Read the model definition and answer for the solid it produces. Units are mm, in the model's axes. A direction names the side the tool comes from. Coordinates: 2 decimals unless noted, no trailing zeros. Order: outer loops, then holes, each group sorted by start corner. A loop starts at its lowest first (then second) coordinate and runs counter-clockwise, first axis right, second up.
```python
from build123d import *

# Parameters (mm, degrees)
SKETCH11_W              = 17
SKETCH11_H              = 19.920243607
BOSS_EXTRUDE7_DEPTH     = 1
BOSS_EXTRUDE5_START     = -2.131780543
BOSS_EXTRUDE5_OUTLINE_W = 1
BOSS_EXTRUDE5_OUTLINE_H = 7
BOSS_EXTRUDE5_DEPTH     = 19.920243607
SKETCH13_W              = 1
SKETCH13_H              = 19.920243607
BOSS_EXTRUDE6_DEPTH     = 7
LPATTERN3_COUNT         = 7
LPATTERN3_PITCH         = 2
CUT_EXTRUDE1_REACH      = 23.276
SKETCH14_R              = 1.905


# Read off the part's stored shape, not the designer's step: Boss-Extrude5
with BuildPart() as part:
    # Sketch11 (on Front Plane) → Boss-Extrude7 (new body)
    with BuildSketch(Plane.XY):
        with Locations((0, 7.828341261)):
            Rectangle(SKETCH11_W, SKETCH11_H)
    extrude(amount=-BOSS_EXTRUDE7_DEPTH)

    # Boss-Extrude5 outline → Boss-Extrude5 (add)
    with BuildSketch(Plane(origin=(0, 0, 0), x_dir=(1, 0, 0), z_dir=(0, 1, 0)).offset(BOSS_EXTRUDE5_START)):
        with Locations((-8, 4.5)):
            Rectangle(BOSS_EXTRUDE5_OUTLINE_W, BOSS_EXTRUDE5_OUTLINE_H)
        with Locations((-8, -3.5)):
            Rectangle(BOSS_EXTRUDE5_OUTLINE_W, BOSS_EXTRUDE5_OUTLINE_H)
    boss_extrude5 = extrude(amount=BOSS_EXTRUDE5_DEPTH)

    # Mirror1: Boss-Extrude5 across plane
    add(boss_extrude5.mirror(Plane(origin=(0, 0, 0), x_dir=(0, 0, 1), z_dir=(1, 0, 0))))

    # Sketch13 → Boss-Extrude6 (add, through all)
    with BuildSketch(Plane(origin=(0, 0, -1), x_dir=(-1, 0, 0), z_dir=(0, 0, -1))):
        with Locations((6, 7.828341261)):
            Rectangle(SKETCH13_W, SKETCH13_H)
    boss_extrude6 = extrude(amount=BOSS_EXTRUDE6_DEPTH)

    # LPattern3: Boss-Extrude6 ×7, 3 skipped
    with Locations(*[(i * LPATTERN3_PITCH, 0, 0) for i in range(1, LPATTERN3_COUNT) if i not in (2, 3, 4)]):
        add(boss_extrude6)

    # Sketch14 → Cut-Extrude1 (cut, up to next)
    with BuildSketch(Plane.XY, mode=Mode.PRIVATE) as cut_extrude1_sk1:
        with Locations((0, 11.468219457)):
            Circle(SKETCH14_R)
    cut_extrude1_tool1 = extrude(cut_extrude1_sk1.sketch, amount=-CUT_EXTRUDE1_REACH, mode=Mode.PRIVATE) & part.part
    add(cut_extrude1_tool1.solids().sort_by_distance((0, 11.468219, 0))[0], mode=Mode.SUBTRACT)


solid = part.part
```
1) Which of the six approach directions +Z, -Z, +X, -X, +Y, -Y give full straight-line access (tool end or side, diameter ignored) to faces 5 (the flat face through (-4, 8, -8)), 6 (the flat face through (-5, 8, -1)), 7 (the flat face through (-7.5, 8, 4))?
A:
face 5: -Z, +X, -X, +Y, -Y
face 6: -Z, +Y, -Y
face 7: +Z, +Y, -Y
2) A cutting plane is placed at D-D, the plane z = 4.5. Determine the outline of the cut face in (x, y), and give its area (3 significant figures).
A:
outline: (-8.5, -2.13) - (-7.5, -2.13) - (-7.5, 17.79) - (-8.5, 17.79) - close; (7.5, -2.13) - (8.5, -2.13) - (8.5, 17.79) - (7.5, 17.79) - close
area: 39.8 mm2
3) Straight lines are drawn through the part: line 1 (X direction, y = 17, z = -3.25); line 2 (X direction, y = 8, z = 5.25); line 3 (Y direction, x = 0, z = -0.55). For each, find the intervals that lie inside material, in ascending order.
A:
line 1: x = -8.5 to -7.5, -6.5 to -5.5, -4.5 to -3.5, 3.5 to 4.5, 5.5 to 6.5, 7.5 to 8.5
line 2: x = -8.5 to -7.5, 7.5 to 8.5
line 3: y = -2.13 to 9.56, 13.37 to 17.79
4) Flat-ended cylindrical pins translate along their axes: pin 1 Ø3.5 at (x, y) = (0, 10) entering from -Z; pin 2 Ø5 at (x, y) = (-2, 8.5) entering from +Z; pin 3 Ø3 at (x, y) = (0, 11.47) entering from +Z. Find the tip coordinate at first contact, or state that the pin passes through.
A:
pin 1: stops at z = -1
pin 2: stops at z = 0
pin 3: passes through
5) Determine the mould class of faces 1 (the flat face through (0, 8, 0)), 2 (the flat face through (-4.5, 8, -4)), 3 (the flat face through (-8.5, 8, 0)), 4 (the flat face through (8.5, 8, 0)) for opening direction X: pulls with the +X half, pulls with the -X half, needs draft (parallel to the pull), parting line crosses it, or undercut.
A:
face 1: undercut
face 2: undercut
face 3: pulls with the -X half
face 4: pulls with the +X half
6) A cutting plane is placed at A-A, the plane z = -6.5. Determine the outline of the cut face in (x, y).
A:
outline: (-8.5, -2.13) - (-7.5, -2.13) - (-7.5, 17.79) - (-8.5, 17.79) - close; (-6.5, -2.13) - (-5.5, -2.13) - (-5.5, 17.79) - (-6.5, 17.79) - close; (-4.5, -2.13) - (-3.5, -2.13) - (-3.5, 17.79) - (-4.5, 17.79) - close; (3.5, -2.13) - (4.5, -2.13) - (4.5, 17.79) - (3.5, 17.79) - close; (5.5, -2.13) - (6.5, -2.13) - (6.5, 17.79) - (5.5, 17.79) - close; (7.5, -2.13) - (8.5, -2.13) - (8.5, 17.79) - (7.5, 17.79) - close
7) A cutting plane is placed at B-B, the plane x = 0. Determine the outline of the cut face in (y, z), and give its area (3 significant figures).
A:
outline: (-2.13, -1) - (9.56, -1) - (9.56, 0) - (-2.13, 0) - close; (13.37, -1) - (17.79, -1) - (17.79, 0) - (13.37, 0) - close
area: 16.1 mm2
